CAD build for the part. Positions are in the model's coordinates, mm. Give positions to 0.01 mm unless a question says otherwise; leave off trailing zeros. Write item = value, one per line. Start each with the question number.
```python
from build123d import *

# Parameters (mm, degrees)
F1_DEPTH = 5.08


# Not quite as in the source:
# - ends of sketch curves that miss each other by under 0.0002 mm in the source are joined


with BuildPart() as f1:
    # F0 (on Front) → F1 (new body)
    with BuildSketch(Plane.XZ):
        with BuildLine():
            add(Edge.make_bspline(
                [(69.85, 59.9050451917), (69.6591630317, 58.0205304518), (69.4657837415, 56.105507858), (69.2658161809, 54.1639224361)],
                knots=[0, 0, 0, 0, 6.3686924223, 6.3686924223, 6.3686924223, 6.3686924223], degree=3))
            add(Edge.make_bspline(
                [(69.85, 59.9050451917), (29.6646114439, 43.1978777051), (22.2865504252, 40.336203924), (0, 54.8465235897)],
                knots=[0, 0, 0, 0, 70.0329289749, 70.0329289749, 70.0329289749, 70.0329289749], degree=3))
            add(Edge.make_bspline(
                [(-69.85, 59.9050451917), (-29.6646114439, 43.1978777051), (-22.2865504252, 40.336203924), (0, 54.8465235897)],
                knots=[0, 0, 0, 0, 70.0329289749, 70.0329289749, 70.0329289749, 70.0329289749], degree=3))
            add(Edge.make_bspline(
                [(-69.85, 59.9050451917), (-69.6591630317, 58.0205304518), (-69.4657837415, 56.105507858), (-69.2658161809, 54.1639224361)],
                knots=[0, 0, 0, 0, 6.3686924223, 6.3686924223, 6.3686924223, 6.3686924223], degree=3))
            add(Edge.make_bspline(
                [(-69.2658161783, 54.1639224373), (-68.435377118, 53.8183422364), (-66.6556116111, 53.0753974425), (-64.8761610511, 52.3317704272), (-63.9263795957, 51.9355805251)],
                knots=[2.7434490873, 2.7434490873, 2.7434490873, 2.7434490873, 5.4418546999, 8.5291588217, 8.5291588217, 8.5291588217, 8.5291588217], degree=3))
            add(Edge.make_bspline(
                [(-63.9263795957, 51.9355805251), (-61.8621309574, 51.0745040519), (-56.1021142689, 48.6812764055), (-47.7406374178, 45.3549636264), (-39.4375160633, 42.5935516843), (-33.4464354817, 41.219419811), (-28.7724481834, 40.4865030944), (-24.7049900131, 40.2576737616), (-20.7256507732, 40.4650803867), (-16.8202071601, 41.130682749), (-12.9707995749, 42.2328724248), (-8.7178720085, 43.9515281326), (-4.3615220824, 46.044445106), (-1.3844475727, 47.8958436146), (-0.0332400038, 48.7623797008), (0, 48.7837122639)],
                knots=[8.5291588217, 8.5291588217, 8.5291588217, 8.5291588217, 15.2390848713, 27.2415659858, 35.5219361762, 41.4579165876, 45.6606303606, 49.7014880209, 53.6563538897, 57.5892253523, 61.5614465465, 65.6429176226, 71.3392641934, 76.0338793574, 76.152307097, 76.152307097, 76.152307097, 76.152307097], degree=3))
            add(Edge.make_bspline(
                [(63.9263795957, 51.9355805251), (61.8621309574, 51.0745040519), (56.1021142689, 48.6812764055), (47.7406374178, 45.3549636264), (39.4375160633, 42.5935516843), (33.4464354817, 41.219419811), (28.7724481834, 40.4865030944), (24.7049900131, 40.2576737616), (20.7256507732, 40.4650803867), (16.8202071601, 41.130682749), (12.9707995749, 42.2328724248), (8.7178720085, 43.9515281326), (4.3615220824, 46.044445106), (1.3844475727, 47.8958436146), (0.0332400038, 48.7623797008), (0, 48.7837122639)],
                knots=[8.5291588217, 8.5291588217, 8.5291588217, 8.5291588217, 15.2390848713, 27.2415659858, 35.5219361762, 41.4579165876, 45.6606303606, 49.7014880209, 53.6563538897, 57.5892253523, 61.5614465465, 65.6429176226, 71.3392641934, 76.0338793574, 76.152307097, 76.152307097, 76.152307097, 76.152307097], degree=3))
            add(Edge.make_bspline(
                [(69.2658161783, 54.1639224373), (68.435377118, 53.8183422364), (66.6556116111, 53.0753974425), (64.8761610511, 52.3317704272), (63.9263795957, 51.9355805251)],
                knots=[2.7434490873, 2.7434490873, 2.7434490873, 2.7434490873, 5.4418546999, 8.5291588217, 8.5291588217, 8.5291588217, 8.5291588217], degree=3))
        make_face()
        with BuildLine():
            add(Edge.make_bspline(
                [(69.2658161809, 54.1639224361), (64.7750418343, 10.5607401093), (56.961539529, -46.4391375943), (0, -72.1534764103)],
                knots=[6.3686924223, 6.3686924223, 6.3686924223, 6.3686924223, 149.3936934001, 149.3936934001, 149.3936934001, 149.3936934001], degree=3))
            add(Edge.make_bspline(
                [(69.2658161809, 54.1639224361), (68.435377118, 53.8183422364), (66.6556116111, 53.0753974425), (64.8761610511, 52.3317704272), (63.9263795957, 51.9355805251)],
                knots=[2.7434490873, 2.7434490873, 2.7434490873, 2.7434490873, 5.4418546999, 8.5291588217, 8.5291588217, 8.5291588217, 8.5291588217], degree=3))
            add(Edge.make_bspline(
                [(63.9263795957, 51.9355805251), (63.6253355549, 49.0777517049), (62.6683683388, 40.3495230581), (60.6243910667, 25.2903357755), (56.8644266428, 6.9882226507), (51.2318594545, -10.9343345603), (43.1811515415, -27.8959051236), (32.1695249216, -43.368046578), (18.0779778329, -56.4464882841), (6.2692486092, -63.5700966147), (1.35086e-05, -66.5543592491)],
                knots=[0.0627067414, 0.0627067414, 0.0627067414, 0.0627067414, 0.125, 0.25, 0.375, 0.5, 0.625, 0.75, 0.875, 0.9876294304, 0.9876294304, 0.9876294304, 0.9876294304], degree=3))
            add(Edge.make_bspline(
                [(-63.9263795983, 51.9355805238), (-63.6253355549, 49.0777517049), (-62.6683683388, 40.3495230581), (-60.6243910667, 25.2903357755), (-56.8644266428, 6.9882226507), (-51.2318594545, -10.9343345603), (-43.1811515415, -27.8959051236), (-32.1695249216, -43.368046578), (-18.0779778329, -56.4464882841), (-6.2692486092, -63.5700966147), (1.35086e-05, -66.5543592491)],
                knots=[0.0627067414, 0.0627067414, 0.0627067414, 0.0627067414, 0.125, 0.25, 0.375, 0.5, 0.625, 0.75, 0.875, 0.9876294304, 0.9876294304, 0.9876294304, 0.9876294304], degree=3))
            add(Edge.make_bspline(
                [(-69.2658161783, 54.1639224373), (-68.435377118, 53.8183422364), (-66.6556116111, 53.0753974425), (-64.8761610511, 52.3317704272), (-63.9263795983, 51.9355805238)],
                knots=[2.7434490873, 2.7434490873, 2.7434490873, 2.7434490873, 5.4418546999, 8.5291588217, 8.5291588217, 8.5291588217, 8.5291588217], degree=3))
            add(Edge.make_bspline(
                [(-69.2658161783, 54.1639224373), (-64.7750418343, 10.5607401093), (-56.961539529, -46.4391375943), (0, -72.1534764103)],
                knots=[6.3686924223, 6.3686924223, 6.3686924223, 6.3686924223, 149.3936934001, 149.3936934001, 149.3936934001, 149.3936934001], degree=3))
        make_face()
        with BuildLine():
            add(Edge.make_bspline(
                [(63.9263795983, 51.9355805238), (63.6253355549, 49.0777517049), (62.6683683388, 40.3495230581), (60.6243910667, 25.2903357755), (56.8644266428, 6.9882226507), (51.2318594545, -10.9343345603), (43.1811515415, -27.8959051236), (32.1695249216, -43.368046578), (18.0779778329, -56.4464882841), (6.2692486092, -63.5700966147), (1.35086e-05, -66.5543592491)],
                knots=[0.0627067414, 0.0627067414, 0.0627067414, 0.0627067414, 0.125, 0.25, 0.375, 0.5, 0.625, 0.75, 0.875, 0.9876294304, 0.9876294304, 0.9876294304, 0.9876294304], degree=3))
            add(Edge.make_bspline(
                [(63.9263795983, 51.9355805238), (61.8621309574, 51.0745040519), (56.1021142689, 48.6812764055), (47.7406374178, 45.3549636264), (39.4375160633, 42.5935516843), (33.4464354817, 41.219419811), (28.7724481834, 40.4865030944), (24.7049900131, 40.2576737616), (20.7256507732, 40.4650803867), (16.8202071601, 41.130682749), (12.9707995749, 42.2328724248), (8.7178720085, 43.9515281326), (4.3615220824, 46.044445106), (1.3844475727, 47.8958436146), (0.0332400038, 48.7623797008), (0, 48.7837122639)],
                knots=[8.5291588217, 8.5291588217, 8.5291588217, 8.5291588217, 15.2390848713, 27.2415659858, 35.5219361762, 41.4579165876, 45.6606303606, 49.7014880209, 53.6563538897, 57.5892253523, 61.5614465465, 65.6429176226, 71.3392641934, 76.0338793574, 76.152307097, 76.152307097, 76.152307097, 76.152307097], degree=3))
            add(Edge.make_bspline(
                [(-63.9263795957, 51.9355805251), (-61.8621309574, 51.0745040519), (-56.1021142689, 48.6812764055), (-47.7406374178, 45.3549636264), (-39.4375160633, 42.5935516843), (-33.4464354817, 41.219419811), (-28.7724481834, 40.4865030944), (-24.7049900131, 40.2576737616), (-20.7256507732, 40.4650803867), (-16.8202071601, 41.130682749), (-12.9707995749, 42.2328724248), (-8.7178720085, 43.9515281326), (-4.3615220824, 46.044445106), (-1.3844475727, 47.8958436146), (-0.0332400038, 48.7623797008), (0, 48.7837122639)],
                knots=[8.5291588217, 8.5291588217, 8.5291588217, 8.5291588217, 15.2390848713, 27.2415659858, 35.5219361762, 41.4579165876, 45.6606303606, 49.7014880209, 53.6563538897, 57.5892253523, 61.5614465465, 65.6429176226, 71.3392641934, 76.0338793574, 76.152307097, 76.152307097, 76.152307097, 76.152307097], degree=3))
            add(Edge.make_bspline(
                [(-63.9263795957, 51.9355805251), (-63.6253355549, 49.0777517049), (-62.6683683388, 40.3495230581), (-60.6243910667, 25.2903357755), (-56.8644266428, 6.9882226507), (-51.2318594545, -10.9343345603), (-43.1811515415, -27.8959051236), (-32.1695249216, -43.368046578), (-18.0779778329, -56.4464882841), (-6.2692486092, -63.5700966147), (1.35086e-05, -66.5543592491)],
                knots=[0.0627067414, 0.0627067414, 0.0627067414, 0.0627067414, 0.125, 0.25, 0.375, 0.5, 0.625, 0.75, 0.875, 0.9876294304, 0.9876294304, 0.9876294304, 0.9876294304], degree=3))
        make_face()
    extrude(amount=F1_DEPTH)


solid = f1.part
```
1. Pin check, flat tips, straight feed: pin 1 Ø2 at (x, z) = (-8.5, -53) entering from +Y; pin 2 Ø1 at (y, z) = (-0.5, -52.5) entering from -X; pin 3 Ø1 at (x, y) = (38.5, -1.5) entering from -Z; pin 4 Ø1 at (y, z) = (-4, -11) entering from +X. Stop position of each tip, or through.
2. Wall check: line 1 along Z through (x, y) = (10.5, -1.95); line 2 along Z through (x, y) = (-13, -1); line 3 along X through (y, z) = (-1.2, 25). Give the ranges that are in metal, low to high.
3. Cut at A-A (z = 49). Count the separate pieces of the cut face and the enclosed holes in it, then the cut area to 3 significant figures.
Output:
q1.pin_1 = 0
q1.pin_2 = -30.04
q1.pin_3 = -43.32
q1.pin_4 = 56.37
q2.line_1 = -66.75 to 48.85
q2.line_2 = -65.25 to 47.78
q2.line_3 = -65.52 to 65.52
q3.separate_pieces = 3
q3.enclosed_holes = 0
q3.area = 373 mm2
